from build123d import *

# Parameters (mm, degrees)
TUBE_SQUARE_40_X_40_X_3_2_1_DEPTH = 2000
CUT_EXTRUDE1_DEPTH                = 2001.499937516
SKETCH17_R                        = 2
CUT_EXTRUDE2_DEPTH                = 3


with BuildPart() as part:
    # Sketch15 → Tube (square) 40 X 40 X 3.2(1) (new body)
    with BuildSketch(Plane(origin=(0, 0, 0), x_dir=(-1, 0, 0), z_dir=(0, 1, 0))):
        with BuildLine():
            Line((-13.6, -20), (13.6, -20))
            ThreePointArc((13.6, -20), (18.1254834, -18.1254834), (20, -13.6))
            Line((20, -13.6), (20, 13.6))
            ThreePointArc((20, 13.6), (18.1254834, 18.1254834), (13.6, 20))
            Line((13.6, 20), (-13.6, 20))
            ThreePointArc((-13.6, 20), (-18.1254834, 18.1254834), (-20, 13.6))
            Line((-20, 13.6), (-20, -13.6))
            ThreePointArc((-20, -13.6), (-18.1254834, -18.1254834), (-13.6, -20))
        make_face()
        with BuildLine():
            Line((-13.6, -16.8), (13.6, -16.8))
            ThreePointArc((13.6, -16.8), (15.8627417, -15.8627417), (16.8, -13.6))
            Line((16.8, -13.6), (16.8, 13.6))
            ThreePointArc((16.8, 13.6), (15.8627417, 15.8627417), (13.6, 16.8))
            Line((13.6, 16.8), (-13.6, 16.8))
            ThreePointArc((-13.6, 16.8), (-15.8627417, 15.8627417), (-16.8, 13.6))
            Line((-16.8, 13.6), (-16.8, -13.6))
            ThreePointArc((-16.8, -13.6), (-15.8627417, -15.8627417), (-13.6, -16.8))
        make_face(mode=Mode.SUBTRACT)
    extrude(amount=TUBE_SQUARE_40_X_40_X_3_2_1_DEPTH)

    # Sketch13 → Cut-Extrude1 (cut, through all)
    with BuildSketch(Plane(origin=(0, 0, -20), x_dir=(-1, 0, 0), z_dir=(0, 0, -1))):
        Polygon((20, 1960), (-20, 2000), (20, 2000), align=None)
        Polygon((-20, 0), (20, 40), (20, 0), align=None)
    extrude(amount=-CUT_EXTRUDE1_DEPTH, mode=Mode.SUBTRACT)

    # Sketch17 → Cut-Extrude2 (cut)
    with BuildSketch(Plane(origin=(20, 0, 0), x_dir=(0, 0, -1), z_dir=(1, 0, 0))):
        with Locations((0, 1980)):
            Circle(SKETCH17_R)
        with Locations((0, 20)):
            Circle(SKETCH17_R)
        with Locations((0, 1020)):
            Circle(SKETCH17_R)
        with Locations((0, 980)):
            Circle(SKETCH17_R)
        with Locations((0, 500)):
            Circle(SKETCH17_R)
        with Locations((0, 1500)):
            Circle(SKETCH17_R)
    extrude(amount=-CUT_EXTRUDE2_DEPTH, mode=Mode.SUBTRACT)


solid = part.part
Work out the finished part from the listing and answer in its coordinate system (mm). Give positions to 0.01 mm unless a question says otherwise; leave off trailing zeros. Loops run counter-clockwise (first coordinate to the right, second up) from the corner with the lowest first, then second, coordinate; pieces in that order, holes last. Notation, with made-up numbers: (35, 7) -> (42, 7) arc R19 ccw to (42, 24) -> close; hole circle Ø7 at (66.5, -14.5). An arc over 180 degrees is marked (long way). Use a Markdown table: item, result. Add a question column.
1) Each of these flat-tipped pins is pushed along its axis until it touches: P1, Ø2.5, axis at y = 1980, z = 0, coming from the -X side; P2, Ø1.2, axis at y = 1979.5, z = 0.5, coming from the +X side; P3, Ø6, axis at x = -14, z = -5, coming from the +Y side. Where does it stop, or does it pass through?
2) The part is cut by section A-A, the plane x = -7.5. Determine the outline of the cut face in (y, z).
3) Consider line 1 along X through (y, z) = (921.5, -7); line 2 along X through (y, z) = (1214.5, 16). Determine where each line is inside the solid, lowest interval first.
4) The part is cut by section B-B, the plane y = 1086. Determine the outline of the cut face in (x, z), plus the area to 3 significant figures.
Reported:
| question | item | result |
|---|---|---|
| 1 | P1 | stops at x = 16.8 |
| 1 | P2 | stops at x = 17 |
| 1 | P3 | stops at y = 1963.2 |
| 2 | outline | (27.5, -20) -> (1972.5, -20) -> (1972.5, -16.8) -> (27.5, -16.8) -> close; (27.5, 16.8) -> (1972.5, 16.8) -> (1972.5, 20) -> (27.5, 20) -> close |
| 3 | line 1 | x = -20 to -16.8, 16.8 to 20 |
| 3 | line 2 | x = -19.53 to -15.72, 15.72 to 19.53 |
| 4 | outline | (-20, -13.6) arc R6.4 ccw to (-13.6, -20) -> (13.6, -20) arc R6.4 ccw to (20, -13.6) -> (20, 13.6) arc R6.4 ccw to (13.6, 20) -> (-13.6, 20) arc R6.4 ccw to (-20, 13.6) -> close; hole (-16.8, -13.6) arc R3.2 ccw to (-13.6, -16.8) -> (13.6, -16.8) arc R3.2 ccw to (16.8, -13.6) -> (16.8, 13.6) arc R3.2 ccw to (13.6, 16.8) -> (-13.6, 16.8) arc R3.2 ccw to (-16.8, 13.6) -> close |
| 4 | area | 445 mm^2 |
